from build123d import *

# Parameters (mm, degrees)
SKETCH1_W                   = 230
SKETCH1_H                   = 65
BOSS_EXTRUDE1_DEPTH         = 2
M2_5_TAPPED_HOLE1_D         = 2.05
M2_5_TAPPED_HOLE1_DEPTH     = 2.5
M2_5_TAPPED_HOLE1_TIP       = 0.615882135
M2_5_TAPPED_HOLE2_D         = 2.05
M2_5_TAPPED_HOLE2_DEPTH     = 6.35
M2_5_TAPPED_HOLE2_TIP       = 0.615882135
SKETCH12_R                  = 4
BOSS_EXTRUDE4_DEPTH         = 20
FILLET1_R                   = 5
M2_5_TAPPED_HOLE3_D         = 2.05
M2_5_TAPPED_HOLE3_DEPTH     = 6.35
M2_5_TAPPED_HOLE3_TIP       = 0.615882135
M2_5_START                  = 2
M2_5_TAPPED_HOLE4_OUTLINE_R = 1.025
M2_5_TAPPED_HOLE4_DEPTH     = 20
M2_5_TAPPED_HOLE4_2_DEPTH   = 17
M2_5_START_2                = 19
M2_5_TAPPED_HOLE4_3_DEPTH   = 11
M2_5_TAPPED_HOLE5_OUTLINE_R = 1.025
M2_5_TAPPED_HOLE5_DEPTH     = 2


# Read off the part's stored shape, not the designer's step: M2.5 Tapped Hole4, M2.5 Tapped Hole5
with BuildPart() as part:
    # Sketch1 → Boss-Extrude1 (new body)
    with BuildSketch(Plane(origin=(0, 0, 0), x_dir=(1, 0, 0), z_dir=(0, 1, 0))):
        with Locations((115, 32.5)):
            Rectangle(SKETCH1_W, SKETCH1_H)
    extrude(amount=BOSS_EXTRUDE1_DEPTH)

    # M2.5 Tapped Hole1
    with Locations(Plane(origin=(0, 0, 0), x_dir=(-1, 0, 0), z_dir=(0, -1, 0))):
        with Locations((-97, 8.54131446), (-97, 57.54131446), (-155, 57.54131446), (-155, 8.54131446)):
            Hole(M2_5_TAPPED_HOLE1_D / 2, depth=M2_5_TAPPED_HOLE1_DEPTH)
            with Locations((0, 0, -(M2_5_TAPPED_HOLE1_DEPTH + M2_5_TAPPED_HOLE1_TIP / 2))):  # 118° drill point
                Cone(0, M2_5_TAPPED_HOLE1_D / 2, M2_5_TAPPED_HOLE1_TIP, mode=Mode.SUBTRACT)

    # M2.5 Tapped Hole2
    with Locations(Plane(origin=(0, 0, 0), x_dir=(-1, 0, 0), z_dir=(0, -1, 0))):
        with Locations((-10, 17.256022479), (-22.3, 17.256022479), (-22.3, 38.056022479), (-10, 38.056022479)):
            Hole(M2_5_TAPPED_HOLE2_D / 2, depth=M2_5_TAPPED_HOLE2_DEPTH)
            with Locations((0, 0, -(M2_5_TAPPED_HOLE2_DEPTH + M2_5_TAPPED_HOLE2_TIP / 2))):  # 118° drill point
                Cone(0, M2_5_TAPPED_HOLE2_D / 2, M2_5_TAPPED_HOLE2_TIP, mode=Mode.SUBTRACT)

    # Sketch12 → Boss-Extrude4 (add)
    with BuildSketch(Plane(origin=(0, 2, 0), x_dir=(1, 0, 0), z_dir=(0, 1, 0))):
        with Locations(Location((10, 38.056022479, 0), (0, 0, 90))):
            Circle(SKETCH12_R)
        with Locations(Location((22.3, 38.056022479, 0), (0, 0, 90))):
            Circle(SKETCH12_R)
        with Locations(Location((10, 17.256022479, 0), (0, 0, 90))):
            Circle(SKETCH12_R)
        with Locations(Location((22.3, 17.256022479, 0), (0, 0, 90))):
            Circle(SKETCH12_R)
    extrude(amount=BOSS_EXTRUDE4_DEPTH)

    # Fillet1
    fillet1_edges = [part.edges().sort_by_distance(p)[0] for p in [
        (0, 1, -65),
        (230, 1, -65),
        (230, 1, 0),
        (0, 1, 0),
    ]]
    fillet(fillet1_edges, radius=FILLET1_R)

    # M2.5 Tapped Hole3
    with Locations(Plane(origin=(5, 0, -5), x_dir=(0, 0, -1), z_dir=(0, -1, 0))):
        with Locations((0, 0), (0, 220), (55, 220), (55, 0)):
            Hole(M2_5_TAPPED_HOLE3_D / 2, depth=M2_5_TAPPED_HOLE3_DEPTH)
            with Locations((0, 0, -(M2_5_TAPPED_HOLE3_DEPTH + M2_5_TAPPED_HOLE3_TIP / 2))):  # 118° drill point
                Cone(0, M2_5_TAPPED_HOLE3_D / 2, M2_5_TAPPED_HOLE3_TIP, mode=Mode.SUBTRACT)

    # M2.5 Tapped Hole4 outline → M2.5 Tapped Hole4 (cut)
    with BuildSketch(Plane(origin=(0, 0, 0), x_dir=(1, 0, 0), z_dir=(0, 1, 0)).offset(M2_5_START)):
        with Locations((10, 38.056022479)):
            Circle(M2_5_TAPPED_HOLE4_OUTLINE_R)
        with Locations((22.3, 38.056022479)):
            Circle(M2_5_TAPPED_HOLE4_OUTLINE_R)
        with Locations((22.3, 17.256022479)):
            Circle(M2_5_TAPPED_HOLE4_OUTLINE_R)
        with Locations((10, 17.256022479)):
            Circle(M2_5_TAPPED_HOLE4_OUTLINE_R)
    extrude(amount=M2_5_TAPPED_HOLE4_DEPTH, mode=Mode.SUBTRACT)

    # M2.5 Tapped Hole4 2 outline → M2.5 Tapped Hole4 2 (add)
    with BuildSketch(Plane(origin=(0, 0, 0), x_dir=(1, 0, 0), z_dir=(0, 1, 0)).offset(M2_5_START)):
        with BuildLine():
            ThreePointArc((211.782562929, 17.990693318), (221.179581033, 22.937725916), (225.985844998, 32.407515116))
            Line((225.985844998, 32.407515116), (223.447313577, 32.407515116))
            ThreePointArc((223.447313577, 32.407515116), (219.412240688, 24.706042811), (211.782562929, 20.536809526))
            Line((211.782562929, 20.536809526), (211.782562929, 17.990693318))
        make_face()
        with BuildLine():
            ThreePointArc((226.030319518, 37.74300987), (221.281519671, 47.396787308), (211.782562929, 52.448157384))
            Line((211.782562929, 52.448157384), (211.782562929, 49.902041176))
            ThreePointArc((211.782562929, 49.902041176), (219.514410141, 45.6278138), (223.499425569, 37.74300987))
            Line((223.499425569, 37.74300987), (226.030319518, 37.74300987))
        make_face()
        with BuildLine():
            ThreePointArc((206.276217111, 52.548907703), (196.36982105, 47.624674517), (191.39614442, 37.74300987))
            Line((191.39614442, 37.74300987), (193.927038369, 37.74300987))
            ThreePointArc((193.927038369, 37.74300987), (198.137709859, 45.857015872), (206.276217111, 50.020133394))
            Line((206.276217111, 50.020133394), (206.276217111, 52.548907703))
        make_face()
        with BuildLine():
            ThreePointArc((191.440618941, 32.407515116), (196.473651384, 22.711721041), (206.276217111, 17.889942999))
            Line((206.276217111, 17.889942999), (206.276217111, 20.418717308))
            ThreePointArc((206.276217111, 20.418717308), (198.242107068, 24.479055557), (193.979150361, 32.407515116))
            Line((193.979150361, 32.407515116), (191.440618941, 32.407515116))
        make_face()
        with BuildLine():
            ThreePointArc((211.782562929, 21.150338406), (218.988116471, 25.13048346), (222.836020675, 32.407515116))
            Line((222.836020675, 32.407515116), (217.262685801, 32.407515116))
            ThreePointArc((217.262685801, 32.407515116), (215.172762854, 28.952491432), (211.782562929, 26.758975749))
            Line((211.782562929, 26.758975749), (211.782562929, 21.150338406))
        make_face()
        with BuildLine():
            ThreePointArc((222.89037982, 37.74300987), (219.090366179, 45.203166413), (211.782562929, 49.288512296))
            Line((211.782562929, 49.288512296), (211.782562929, 43.679874952))
            ThreePointArc((211.782562929, 43.679874952), (215.276963699, 41.377138058), (217.352185678, 37.74300987))
            Line((217.352185678, 37.74300987), (222.89037982, 37.74300987))
        make_face()
        with BuildLine():
            ThreePointArc((206.276217111, 49.411710529), (198.562013106, 45.432786972), (194.536084119, 37.74300987))
            Line((194.536084119, 37.74300987), (200.074278261, 37.74300987))
            ThreePointArc((200.074278261, 37.74300987), (202.381190604, 41.615146745), (206.276217111, 43.883198119))
            Line((206.276217111, 43.883198119), (206.276217111, 49.411710529))
        make_face()
        with BuildLine():
            ThreePointArc((194.590443263, 32.407515116), (198.666590392, 24.903176371), (206.276217111, 21.027140173))
            Line((206.276217111, 21.027140173), (206.276217111, 26.555652583))
            ThreePointArc((206.276217111, 26.555652583), (202.489350756, 28.718402151), (200.163778137, 32.407515116))
            Line((200.163778137, 32.407515116), (194.590443263, 32.407515116))
        make_face()
    extrude(amount=M2_5_TAPPED_HOLE4_2_DEPTH)

    # M2.5 Tapped Hole4 3 outline → M2.5 Tapped Hole4 3 (add)
    with BuildSketch(Plane(origin=(0, 0, 0), x_dir=(1, 0, 0), z_dir=(0, 1, 0)).offset(M2_5_START_2)):
        with BuildLine():
            ThreePointArc((211.782562929, 17.990693318), (221.179581033, 22.937725916), (225.985844998, 32.407515116))
            Line((225.985844998, 32.407515116), (223.447313577, 32.407515116))
            ThreePointArc((223.447313577, 32.407515116), (219.412240688, 24.706042811), (211.782562929, 20.536809526))
            Line((211.782562929, 20.536809526), (211.782562929, 17.990693318))
        make_face()
        with BuildLine():
            ThreePointArc((226.030319518, 37.74300987), (221.281519671, 47.396787308), (211.782562929, 52.448157384))
            Line((211.782562929, 52.448157384), (211.782562929, 49.902041176))
            ThreePointArc((211.782562929, 49.902041176), (219.514410141, 45.6278138), (223.499425569, 37.74300987))
            Line((223.499425569, 37.74300987), (226.030319518, 37.74300987))
        make_face()
        with BuildLine():
            ThreePointArc((206.276217111, 52.548907703), (196.36982105, 47.624674517), (191.39614442, 37.74300987))
            Line((191.39614442, 37.74300987), (193.927038369, 37.74300987))
            ThreePointArc((193.927038369, 37.74300987), (198.137709859, 45.857015872), (206.276217111, 50.020133394))
            Line((206.276217111, 50.020133394), (206.276217111, 52.548907703))
        make_face()
        with BuildLine():
            ThreePointArc((191.440618941, 32.407515116), (196.473651384, 22.711721041), (206.276217111, 17.889942999))
            Line((206.276217111, 17.889942999), (206.276217111, 20.418717308))
            ThreePointArc((206.276217111, 20.418717308), (198.242107068, 24.479055557), (193.979150361, 32.407515116))
            Line((193.979150361, 32.407515116), (191.440618941, 32.407515116))
        make_face()
    extrude(amount=M2_5_TAPPED_HOLE4_3_DEPTH)

    # M2.5 Tapped Hole5 outline → M2.5 Tapped Hole5 (cut)
    with BuildSketch(Plane(origin=(0, 0, 0), x_dir=(1, 0, 0), z_dir=(0, 1, 0))):
        with Locations((79.821651761, 49.876027086)):
            Circle(M2_5_TAPPED_HOLE5_OUTLINE_R)
        with Locations((59.821651761, 49.876027086)):
            Circle(M2_5_TAPPED_HOLE5_OUTLINE_R)
    extrude(amount=M2_5_TAPPED_HOLE5_DEPTH, mode=Mode.SUBTRACT)


solid = part.part
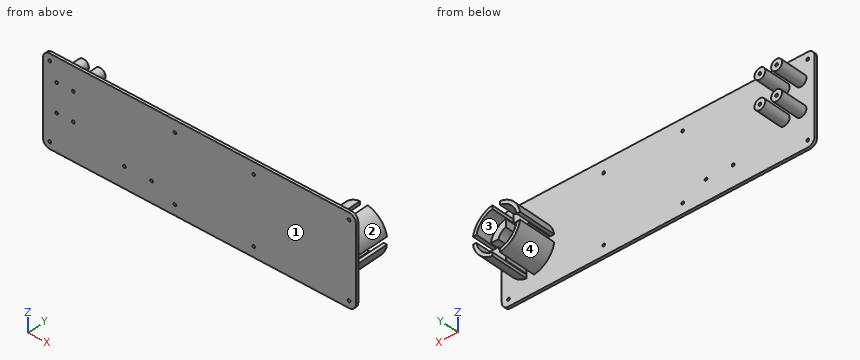
Can you work these out from the model? Positions are in its coordinate system, mm. Face numbers are marked on the shaded views. Give positions to 0.01 mm unless a question says otherwise; leave off trailing zeros. Order: outer loops, then holes, each group sorted by start corner. A loop starts at its lowest first (then second) coordinate and runs counter-clockwise, first axis right, second up. Notation, with made-up numbers: M 26,36 L 76,36 A32 cw 76,72 Z; hole C 41,-28.75 d10. An arc over 180 degrees is marked long. One line per item, written item: value.
Item 1: Please list where these lines run through material, in increasing order: line 1 (Z direction, x = 10, y = 1.4); line 2 (Z direction, x = 97, y = 1.25); line 3 (Z direction, x = 22.3, y = 7).
Verdict:
line 1: -65 to -39.08, -37.03 to -18.28, -16.23 to 0
line 2: -65 to -58.57, -56.52 to -9.57, -7.52 to 0
line 3: -42.06 to -39.08, -37.03 to -34.06, -21.26 to -18.28, -16.23 to -13.26
Item 2: For pin 1 (3 mm diameter, centred on x = 197, y = 7.5, fed in from +Z); pin 2 (12 mm diameter, centred on x = 170.5, z = -25.5, fed in from +Y); pin 3 (2.5 mm diameter, centred on x = 22.3, z = -38.06, fed in from +Y); pin 4 (1.2 mm diameter, centred on x = 97, z = -8.54, fed in from -Y), each with a flat end and sliding along its axis, tell me the tip position at first contact or that it passes through.
Verdict:
pin 1: z = -21.01
pin 2: y = 2
pin 3: y = 22
pin 4: through
Item 3: If we section it at A-A on y = 6.5: State how many separate pieces and enclosed holes the cut face has, and give its area (3 significant figures).
Verdict:
separate pieces: 12
enclosed holes: 4
area: 667 mm2
Item 4: If we section it at B-B on x = 70: Write out the boundary of the cut face in (y, z).
Verdict:
outline: M 0,-65 L 2,-65 L 2,0 L 0,0 Z
Item 5: If we mould it in two halves opening along Z, with no side actions, what happens to the marked faces 1, 2, 3 and 4? For each: pulls with the +Z half, pulls with the -Z half, needs draft (parallel to the pull), parting line crosses it, or undercut.
Verdict:
face 1: needs draft
face 2: pulls with the +Z half
face 3: undercut
face 4: pulls with the -Z half
